from build123d import *

# Parameters (mm, degrees)
F2_SIZE  = 0.5
F5_R     = 9
F5_R_2   = 5.5
F6_DEPTH = 2
F7_R     = 9
F7_R_2   = 5.5
F8_DEPTH = 2


with BuildPart() as f1:
    # F0 (on Right) → F1 (revolve)
    with BuildSketch(Plane.YZ):
        with BuildLine():
            Line((-3.5, 10.5), (-3.5, 4))
            Line((-3.5, 4), (3.5, 4))
            Line((3.5, 4), (3.5, 10.5))
            ThreePointArc((3.5, 10.5), (3.353553, 10.853553), (3, 11))
            Line((3, 11), (-3, 11))
            ThreePointArc((-3, 11), (-3.353553, 10.853553), (-3.5, 10.5))
        make_face()
    revolve(axis=Axis((0, 1.946479, 0), (0, 1, 0)))

    # F2
    f2_edges = [f1.edges().sort_by_distance(p)[0] for p in [
        (0, 3.5, -4),
        (0, -3.5, -4),
    ]]
    chamfer(f2_edges, length=F2_SIZE)

    # F5 (on offset) → F6 (cut)
    with BuildSketch(Plane.XZ.offset(-5)):
        Circle(F5_R)
        Circle(F5_R_2, mode=Mode.SUBTRACT)
    extrude(amount=F6_DEPTH, mode=Mode.SUBTRACT)

    # F7 (on offset) → F8 (cut)
    with BuildSketch(Plane.XZ.offset(5)):
        Circle(F7_R)
        Circle(F7_R_2, mode=Mode.SUBTRACT)
    extrude(amount=-F8_DEPTH, mode=Mode.SUBTRACT)


solid = f1.part
CAD build for the part. Positions are in the model's coordinates, mm. A direction names the side the tool comes from. Round coordinates to 2 decimals unless told otherwise and drop trailing zeros. Loops run counter-clockwise (first coordinate to the right, second up) from the corner with the lowest first, then second, coordinate; pieces in that order, holes last. Notation, with made-up numbers: M 45.25,0 L 65.25,0 A18 cw 65.25,23 Z; hole C 68.25,58 d11. An arc over 180 degrees is marked long. One line per question, with ' | ' between items. Start each with the question number.
Item 1: Which spindle directions (+Z, -Z, +X, -X, +Y, -Y) get a long thin tool onto all of the face, cutting with end or side? Do faces 4 (the cylindrical face through (-1.19, -3.25, -5.37)), 5 (the flat face through (-4, 3, -4)), 6 (the cylindrical face through (-3.905, 0.042, -0.867)). Say none if no direction does.
Item 2: Two-plate mould, pull along X, no slides. Class faces 1 (the cylindrical face through (-10.74, -0.04, -2.38)), 2 (the flat face through (5, -3.5, 8)), 3 (the flat face through (-4, -3, -4)): pulls with the +X half, pulls with the -X half, needs draft (parallel to the pull), parting line crosses it, or undercut.
Item 3: Cut at C-C, the plane y = -1.5. Write the cut outline in (x, z).
Item 4: Wall check: line 1 (X direction, y = 3.2, z = 0); line 2 (Y direction, x = -5.5, z = -3.5); line 3 (X direction, y = 0, z = 3.5). Give the ranges that are in metal, low to high.
Item 5: Pin check, flat tips, straight feed: pin 1 Ø1 at (x, y) = (8.5, -1) entering from +Z; pin 2 Ø1 at (x, z) = (-3, 5.5) entering from +Y; pin 3 Ø2 at (x, y) = (-3.5, 1.5) entering from +Z. Stop position of each tip, or through.
Responses:
1) face 4: -Y | face 5: +Y | face 6: +Y, -Y
2) face 1: parting line crosses it | face 2: needs draft | face 3: undercut
3) outline: C 0,0 d22; hole C 0,0 d8
4) line 1: x = -10.96 to -9, -5.5 to -4.2, 4.2 to 5.5, 9 to 10.96 | line 2: y = -3 to 3 | line 3: x = -10.43 to -1.94, 1.94 to 10.43
5) pin 1: stops at z = 7.55 | pin 2: stops at y = 3 | pin 3: stops at z = 10.71
